```python
from build123d import *

# Parameters (mm, degrees)
SKETCH1_W           = 203.2
SKETCH1_H           = 215.9
BOSS_EXTRUDE1_DEPTH = 213.36
SHELL2_T            = -12.7
SKETCH2_W           = 76.2
SKETCH2_H           = 76.2
CUT_EXTRUDE1_DEPTH  = 6.35
SKETCH3_R           = 6.35
CUT_EXTRUDE2_DEPTH  = 250.479855099
CUT_EXTRUDE3_DEPTH  = 314.792817158


with BuildPart() as part:
    # Sketch1 → Boss-Extrude1 (new body)
    with BuildSketch(Plane(origin=(0, 0, 0), x_dir=(1, 0, 0), z_dir=(0, 1, 0))):
        Rectangle(SKETCH1_W, SKETCH1_H)
    extrude(amount=BOSS_EXTRUDE1_DEPTH)

    # Shell2
    shell2_openings = [part.faces().sort_by_distance(p)[0] for p in [
        (0, 213.36, 0),
        (0, 106.68, 107.95),
    ]]
    offset(amount=SHELL2_T, openings=shell2_openings, kind=Kind.INTERSECTION)

    # Sketch2 → Cut-Extrude1 (cut)
    with BuildSketch(Plane(origin=(0, 12.7, 0), x_dir=(1, 0, 0), z_dir=(0, 1, 0))):
        Rectangle(SKETCH2_W, SKETCH2_H)
    extrude(amount=-CUT_EXTRUDE1_DEPTH, mode=Mode.SUBTRACT)

    # Sketch3 → Cut-Extrude2 (cut, through all)
    with BuildSketch(Plane(origin=(0, 12.7, 0), x_dir=(1, 0, 0), z_dir=(0, 1, 0))):
        with Locations(Location((-76.2, 63.5, 0), (0, 0, 270))):
            Circle(SKETCH3_R)
        with Locations(Location((-76.2, -63.5, 0), (0, 0, 270))):
            Circle(SKETCH3_R)
        with Locations(Location((76.2, 63.5, 0), (0, 0, 270))):
            Circle(SKETCH3_R)
        with Locations(Location((76.2, -63.5, 0), (0, 0, 270))):
            Circle(SKETCH3_R)
    extrude(amount=-CUT_EXTRUDE2_DEPTH, mode=Mode.SUBTRACT)

    # Sketch4 → Cut-Extrude3 (cut, through all)
    with BuildSketch(Plane(origin=(101.6, 0, 0), x_dir=(0, 0, -1), z_dir=(1, 0, 0))):
        Polygon((48.42184808, 213.36), (-107.95, 0), (-107.95, 213.36), align=None)
    extrude(amount=-CUT_EXTRUDE3_DEPTH, mode=Mode.SUBTRACT)


solid = part.part
```
Design review of the part built by this model. Coordinates are the model's own, in mm. A direction names the side the tool comes from. Give positions to 0.01 mm unless a question says otherwise; leave off trailing zeros. Loops run counter-clockwise (first coordinate to the right, second up) from the corner with the lowest first, then second, coordinate; pieces in that order, holes last. Notation, with made-up numbers: (77.25, 83) -> (119.25, 83) arc R16 ccw to (119.25, 96) -> close; hole circle Ø6 at (55.5, 78). An arc over 180 degrees is marked (long way). Write each question's results on one line, items separated by ' | '.
Q1. Take a section at A-A, the plane x = 76.2. Write out the cut boundary in (y, z).
Reply:
outline: (0, -107.95) -> (213.36, -107.95) -> (213.36, -95.25) -> (12.7, -95.25) -> (12.7, -69.85) -> (0, -69.85) -> close; (0, -57.15) -> (12.7, -57.15) -> (12.7, 57.15) -> (0, 57.15) -> close; (0, 69.85) -> (12.7, 69.85) -> (12.7, 98.64) -> (0, 107.95) -> close
Q2. Machinability: for faces 4 (the face through (38.1, 10, 1)), 5 (the face through (-88.9, 89, -18)), 6 (the face through (-1, 0, -2)), which of the approach directions +Z, -Z, +X, -X, +Y, -Y give a long, thin tool a straight path to every point of the face, cutting with its end or side? Answer none if there is none.
Reply:
face 4: +Y | face 5: +Z, +Y | face 6: +Z, -Z, +X, -X, -Y
Q3. Take a section at C-C, the plane x = 8.5. Write out the cut boundary in (y, z), plus the area to 3 significant figures.
Reply:
outline: (0, -107.95) -> (213.36, -107.95) -> (213.36, -95.25) -> (12.7, -95.25) -> (12.7, -38.1) -> (6.35, -38.1) -> (6.35, 38.1) -> (12.7, 38.1) -> (12.7, 98.64) -> (0, 107.95) -> close | area: 4,750 mm²
Q4. Wall thickness on L1, parallel to X at y = 9, z = 63.5; L2, parallel to X at y = 160.5, z = -88.5; L3, parallel to Z at x = 76, y = 4: over which ranges is each line inside the solid? List them lowest first.
Reply:
L1: x = -101.6 to -82.55, -69.85 to 69.85, 82.55 to 101.6 | L2: x = -101.6 to -88.9, 88.9 to 101.6 | L3: z = -107.95 to -69.85, -57.15 to 57.15, 69.85 to 105.02
Q5. Take a section at D-D, the plane y = 26. Write out the cut boundary in (x, z).
Reply:
outline: (-101.6, -107.95) -> (101.6, -107.95) -> (101.6, 88.89) -> (88.9, 88.89) -> (88.9, -95.25) -> (-88.9, -95.25) -> (-88.9, 88.89) -> (-101.6, 88.89) -> close
Q6. The part is to be moulded in two halves that separate along Z. For faces 1 (the face through (88.9, 89, -18)), 2 (the face through (-1, 105, -107.95)), 3 (the face through (81.554, 6.439, 66.914)), say which applies: +Z half, -Z half, draft (parallel to the pull), parting line (faces both ways), or undercut.
Reply:
face 1: draft | face 2: -Z half | face 3: undercut
Q7. For pin 1 Ø6 at (x, y) = (-52.5, 129) entering from +Z; pin 2 Ø3 at (x, y) = (16.5, 8) entering from +Z; pin 3 Ø6 at (x, z) = (73.5, 53.5) entering from +Y, all flat-tipped, find the tip position at first contact; note any pin that passes through.
Reply:
pin 1: stops at z = -95.25 | pin 2: stops at z = 103.19 | pin 3: stops at y = 12.7
Q8. Take a section at B-B, the plane z = 63.5. Write out the cut boundary in (x, y).
Reply:
outline: (-101.6, 0) -> (-82.55, 0) -> (-82.55, 12.7) -> (-88.9, 12.7) -> (-88.9, 60.65) -> (-101.6, 60.65) -> close; (-69.85, 0) -> (69.85, 0) -> (69.85, 12.7) -> (-69.85, 12.7) -> close; (82.55, 0) -> (101.6, 0) -> (101.6, 60.65) -> (88.9, 60.65) -> (88.9, 12.7) -> (82.55, 12.7) -> close
